from build123d import *

# Parameters (mm, degrees)
F0_W      = 31
F0_H      = 33
F1_DEPTH  = 2
F2_R      = 3
F3_DEPTH  = 2.4
F4_W      = 16.4
F4_H      = 31
F5_DEPTH  = 1
F6_R      = 1.5
F7_DEPTH  = 3.4
F8_R      = 1.5
F9_DEPTH  = 3.4
F10_R     = 7
F11_DEPTH = 25
F12_DEPTH = 1
F13_W     = 44
F13_H     = 44
F13_W_2   = 31
F13_H_2   = 33
F13_R     = 7
F14_DEPTH = 0.5
F15_R     = 1


with BuildPart() as f1:
    # F0 (on Top) → F1 (new body)
    with BuildSketch(Plane.XY):
        with Locations((15.5, 16.5)):
            Rectangle(F0_W, F0_H)
    extrude(amount=F1_DEPTH)

    # F2 (on face) → F3 (join)
    with BuildSketch(Plane.XY.offset(2)):
        with Locations((4, 3)):
            Circle(F2_R)
        with Locations((4, 26.5)):
            Circle(F2_R)
        with Locations((27, 26.5)):
            Circle(F2_R)
        with Locations((27, 3)):
            Circle(F2_R)
    extrude(amount=F3_DEPTH)

    # F4 (on face) → F5 (cut)
    with BuildSketch(Plane.XY.offset(2)):
        with Locations((15.5, 16.5)):
            Rectangle(F4_W, F4_H)
    extrude(amount=-F5_DEPTH, mode=Mode.SUBTRACT)

    # F6 (on face) → F7 (cut)
    with BuildSketch(Plane.XY.offset(4.4)):
        with Locations((27, 26.5)):
            Circle(F6_R)
    extrude(amount=-F7_DEPTH, mode=Mode.SUBTRACT)

    # F8 (on face) → F9 (cut)
    with BuildSketch(Plane.XY.offset(4.4)):
        with Locations((4, 26.5)):
            Circle(F8_R)
        with Locations((4.0643862449, 2.8885749634)):
            Circle(F8_R)
        with Locations((27.0567759871, 3.0037942342)):
            Circle(F8_R)
    extrude(amount=-F9_DEPTH, mode=Mode.SUBTRACT)

    # F10 (on face) → F11 (cut)
    with BuildSketch(Plane.XY.offset(1)):
        with Locations((15.5, 18.8)):
            Circle(F10_R)
    extrude(amount=-F11_DEPTH, mode=Mode.SUBTRACT)

    # F12 (add): a face of the model
    f12_faces = [f1.faces().sort_by_distance(p)[0] for p in [
        (0.4527692569, 16.5, 0),
    ]]
    extrude(f12_faces, amount=F12_DEPTH)

    # F13 (on face) → F14 (join)
    with BuildSketch(Plane(origin=(0, 0, -1), x_dir=(1, 0, 0), z_dir=(0, 0, -1))):
        with Locations((15.5, -16.5)):
            Rectangle(F13_W, F13_H)
        with Locations((15.5, -16.5)):
            Rectangle(F13_W_2, F13_H_2, mode=Mode.SUBTRACT)
        with Locations((15.5, -16.5)):
            Rectangle(F13_W_2, F13_H_2)
        with Locations((15.5, -18.8)):
            Circle(F13_R, mode=Mode.SUBTRACT)
    extrude(amount=F14_DEPTH)

    # F15
    f15_edges = [f1.edges().sort_by_distance(p)[0] for p in [
        (-6.5, -5.5, -1.25),
        (37.5, -5.5, -1.25),
        (37.5, 38.5, -1.25),
        (-6.5, 38.5, -1.25),
    ]]
    fillet(f15_edges, radius=F15_R)


solid = f1.part
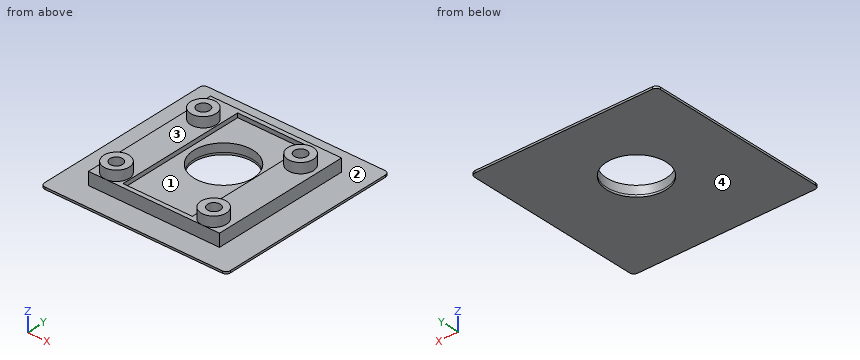
The model under review builds one solid part; all positions refer to its coordinate system, in mm. Face numbers are marked on the shaded views. A direction names the side the tool comes from. Coordinates: 2 decimals unless noted, no trailing zeros. Write each loop counter-clockwise with the first axis right and the second up, starting at its lowest first coordinate (ties: lowest second). Pieces come first, ordered by that corner, then holes. Notation, with made-up numbers: (49, -14.75) - (58, -14.75) arc R17 cw to (58, 1.25) - close; hole circle Ø2 at (-13, -28.5). An arc over 180 degrees is marked (long way). Answer as CSV lines item,"result".
(1) We need section C-C (z = 3.75). Give the boundary of the cut face in (x, y).
Data:
outline,"circle Ø6 at (4, 3); circle Ø6 at (4, 26.5); circle Ø6 at (27, 3); circle Ø6 at (27, 26.5); hole circle Ø3 at (4, 26.5); hole circle Ø3 at (4.06, 2.89); hole circle Ø3 at (27, 26.5); hole circle Ø3 at (27.06, 3)"
(2) We need section A-A (x = 15.5). Give the boundary of the cut face in (y, z).
Data:
outline,"(-5.5, -1.5) - (11.8, -1.5) - (11.8, 1) - (1, 1) - (1, 2) - (0, 2) - (0, -1) - (-5.5, -1) - close; (25.8, -1.5) - (38.5, -1.5) - (38.5, -1) - (33, -1) - (33, 2) - (32, 2) - (32, 1) - (25.8, 1) - close"
(3) Tool access review of the marked faces 3 and 4: name each direction out of +Z, -Z, +X, -X, +Y, -Y from which nothing blocks a thin tool from reaching the whole face with its end or side.
Data:
face 3,"+Z"
face 4,"-Z, +X, -X, +Y, -Y"
(4) We need section B-B (y = 18.8). Give the boundary of the cut face in (x, z).
Data:
outline,"(-6.5, -1.5) - (8.5, -1.5) - (8.5, 1) - (7.3, 1) - (7.3, 2) - (0, 2) - (0, -1) - (-6.5, -1) - close; (22.5, -1.5) - (37.5, -1.5) - (37.5, -1) - (31, -1) - (31, 2) - (23.7, 2) - (23.7, 1) - (22.5, 1) - close"
(5) For line 1 along Y through (x, z) = (15.5, -1.2); line 2 along X through (y, z) = (2, 1.35); line 3 along Z through (x, y) = (24, 9.5), list the stretches that pass through material, from the lowest coordinate up. Write a range as [from, to].
Data:
line 1,"y = [-5.5, 11.8], [25.8, 38.5]"
line 2,"x = [0, 2.86], [5.27, 7.3], [23.7, 25.94], [28.17, 31]"
line 3,"z = [-1.5, 2]"
(6) Mouldability with a two-part tool opening along Y and no side actions: class the marked faces 1 and 2 as pulls with the +Y half, pulls with the -Y half, needs draft (parallel to the pull), parting line crosses it, or undercut.
Data:
face 1,"undercut"
face 2,"needs draft"
(7) Clearance check with flat-ended pins moving along their axes: pin 1 Ø0.9 at (x, y) = (4, 3) entering from +Z; pin 2 Ø0.5 at (x, z) = (15.5, 1.5) entering from -Y; pin 3 Ø8.5 at (x, y) = (15.5, 18.8) entering from +Z; pin 4 Ø15.5 at (x, y) = (17, 18.5) entering from +Z. State where each tip first meets the part, or that it passes through.
Data:
pin 1,"stops at z = 1"
pin 2,"stops at y = 0"
pin 3,"passes through"
pin 4,"stops at z = 2"
(8) We need section D-D (z = 0.15). Give the boundary of the cut face in (x, y).
Data:
outline,"(0, 0) - (31, 0) - (31, 33) - (0, 33) - close; hole circle Ø14 at (15.5, 18.8)"
